from build123d import *

# Parameters (mm, degrees)
SKETCH2_W           = 38.1
SKETCH2_H           = 25.4
SKETCH2_W_2         = 31.75
SKETCH2_H_2         = 19.05
BOSS_EXTRUDE1_DEPTH = 1371.6
CUT_EXTRUDE1_REACH  = 1373.967
SKETCH3_R           = 2.413
CUT_EXTRUDE2_REACH  = 1373.967
SKETCH4_R           = 2.413


with BuildPart() as part:
    # Sketch2 → Boss-Extrude1 (new body)
    with BuildSketch(Plane(origin=(0, 0, 0), x_dir=(1, 0, 0), z_dir=(0, 1, 0))):
        Rectangle(SKETCH2_W, SKETCH2_H)
        Rectangle(SKETCH2_W_2, SKETCH2_H_2, mode=Mode.SUBTRACT)
    extrude(amount=BOSS_EXTRUDE1_DEPTH)

    # Cut-Extrude1: up to this face of the body (flat: up to its plane)
    cut_extrude1_end = Plane(part.part.faces().sort_by_distance((0, 685.8, -12.7))[0])
    # Sketch3 → Cut-Extrude1 (cut, up to the picked face)
    with BuildSketch(Plane.XY.offset(12.7), mode=Mode.PRIVATE) as cut_extrude1_sk1:
        with Locations((0, 31.75)):
            Circle(SKETCH3_R)
    cut_extrude1_tool1 = split(extrude(cut_extrude1_sk1.sketch, amount=-CUT_EXTRUDE1_REACH, mode=Mode.PRIVATE), bisect_by=cut_extrude1_end, keep=Keep.BOTH, mode=Mode.PRIVATE)
    # Sketch3 → Cut-Extrude1 (cut, up to the picked face)
    with BuildSketch(Plane.XY.offset(12.7), mode=Mode.PRIVATE) as cut_extrude1_sk2:
        with Locations((0, 222.25)):
            Circle(SKETCH3_R)
    cut_extrude1_tool2 = split(extrude(cut_extrude1_sk2.sketch, amount=-CUT_EXTRUDE1_REACH, mode=Mode.PRIVATE), bisect_by=cut_extrude1_end, keep=Keep.BOTH, mode=Mode.PRIVATE)
    # Sketch3 → Cut-Extrude1 (cut, up to the picked face)
    with BuildSketch(Plane.XY.offset(12.7), mode=Mode.PRIVATE) as cut_extrude1_sk3:
        with Locations((0, 95.25)):
            Circle(SKETCH3_R)
    cut_extrude1_tool3 = split(extrude(cut_extrude1_sk3.sketch, amount=-CUT_EXTRUDE1_REACH, mode=Mode.PRIVATE), bisect_by=cut_extrude1_end, keep=Keep.BOTH, mode=Mode.PRIVATE)
    add(cut_extrude1_tool1.solids().sort_by(Axis((0, 31.75, 12.7), (0, 0, -1)))[0], mode=Mode.SUBTRACT)
    add(cut_extrude1_tool2.solids().sort_by(Axis((0, 222.25, 12.7), (0, 0, -1)))[0], mode=Mode.SUBTRACT)
    add(cut_extrude1_tool3.solids().sort_by(Axis((0, 95.25, 12.7), (0, 0, -1)))[0], mode=Mode.SUBTRACT)

    # Cut-Extrude2: up to this face of the body (flat: up to its plane)
    cut_extrude2_end = Plane(part.part.faces().sort_by_distance((0, 686.398541634, -12.7))[0])
    # Sketch4 → Cut-Extrude2 (cut, up to the picked face)
    with BuildSketch(Plane.XY.offset(12.7), mode=Mode.PRIVATE) as cut_extrude2_sk1:
        with Locations((0, 1346.2)):
            Circle(SKETCH4_R)
    cut_extrude2_tool1 = split(extrude(cut_extrude2_sk1.sketch, amount=-CUT_EXTRUDE2_REACH, mode=Mode.PRIVATE), bisect_by=cut_extrude2_end, keep=Keep.BOTH, mode=Mode.PRIVATE)
    # Sketch4 → Cut-Extrude2 (cut, up to the picked face)
    with BuildSketch(Plane.XY.offset(12.7), mode=Mode.PRIVATE) as cut_extrude2_sk2:
        with Locations((0, 1320.8)):
            Circle(SKETCH4_R)
    cut_extrude2_tool2 = split(extrude(cut_extrude2_sk2.sketch, amount=-CUT_EXTRUDE2_REACH, mode=Mode.PRIVATE), bisect_by=cut_extrude2_end, keep=Keep.BOTH, mode=Mode.PRIVATE)
    add(cut_extrude2_tool1.solids().sort_by(Axis((0, 1346.2, 12.7), (0, 0, -1)))[0], mode=Mode.SUBTRACT)
    add(cut_extrude2_tool2.solids().sort_by(Axis((0, 1320.8, 12.7), (0, 0, -1)))[0], mode=Mode.SUBTRACT)


solid = part.part
Work out the finished part from the listing and answer in its coordinate system (mm). A direction names the side the tool comes from. Round coordinates to 2 decimals unless told otherwise and drop trailing zeros. Loops run counter-clockwise (first coordinate to the right, second up) from the corner with the lowest first, then second, coordinate; pieces in that order, holes last. Notation, with made-up numbers: (80, 88) - (129, 88) arc R23 ccw to (129, 127) - close; hole circle Ø11 at (-7, -4.75). An arc over 180 degrees is marked (long way). Use one line per item in the form item = value. Start each with the question number.
(1) Which of the six approach directions +Z, -Z, +X, -X, +Y, -Y give full straight-line access (tool end or side, diameter ignored) to faces 1 (the face through (0, 676, -12.7)), 2 (the face through (0, 676, -9.525))?
(2) Find section A-A on x = 8.5. Determine the outline of the cut face in (y, z) (3 decimals).
(3) Flat-ended cylindrical pins translate along their axes: P1, Ø7.5, axis at x = 0, y = 95.25, coming from the +Z side; P2, Ø3, axis at x = 0, y = 1346.2, coming from the -Z side. Find the tip coordinate at first contact, or state that the pin passes through.
(4) Consider line 1 (Y direction, x = 0, z = -11.7); line 2 (X direction, y = 1027, z = 1.5) (3 decimals); line 3 (X direction, y = 1346.2, z = -11.7). Determine where each line is inside the solid, lowest interval first.
(5) Determine the mould class of faces 3 (the face through (19.05, 676, 0)), 4 (the face through (0, 676, 9.525)), 5 (the face through (-19.05, 676, 0)), 6 (the face through (0, 676, 12.7)) for opening direction X: +X half, -X half, draft (parallel to the pull), parting line (faces both ways), or undercut.
(6) Find section C-C on y = 1200. Determine the outline of the cut face in (x, z) (3 decimals).
(7) Find section B-B on z = -4.5. Determine the outline of the cut face in (x, y) (3 decimals).
Answer list:
q1.face_1 = -Z, +X, -X, +Y, -Y
q1.face_2 = +Y, -Y
q2.outline = (0, -12.7) - (1371.6, -12.7) - (1371.6, -9.525) - (0, -9.525) - close; (0, 9.525) - (1371.6, 9.525) - (1371.6, 12.7) - (0, 12.7) - close
q3.P1 = 12.7
q3.P2 = through
q4.line_1 = 0 to 29.34, 34.16 to 92.84, 97.66 to 219.84, 224.66 to 1318.39, 1323.21 to 1343.79, 1348.61 to 1371.6
q4.line_2 = -19.05 to -15.875, 15.875 to 19.05
q4.line_3 = -19.05 to -2.41, 2.41 to 19.05
q5.face_3 = +X half
q5.face_4 = undercut
q5.face_5 = -X half
q5.face_6 = draft
q6.outline = (-19.05, -12.7) - (19.05, -12.7) - (19.05, 12.7) - (-19.05, 12.7) - close; hole (-15.875, -9.525) - (15.875, -9.525) - (15.875, 9.525) - (-15.875, 9.525) - close
q7.outline = (-19.05, 0) - (-15.875, 0) - (-15.875, 1371.6) - (-19.05, 1371.6) - close; (15.875, 0) - (19.05, 0) - (19.05, 1371.6) - (15.875, 1371.6) - close
